Could you check a few things on this model? Use its own coordinates, in mm. Face numbers are marked on the shaded views. A direction names the side the tool comes from. Round coordinates to 2 decimals unless told otherwise and drop trailing zeros. Loops run counter-clockwise (first coordinate to the right, second up) from the corner with the lowest first, then second, coordinate; pieces in that order, holes last. Notation, with made-up numbers: (45.5, 53) -> (96.5, 53) arc R20 ccw to (96.5, 63) -> close; hole circle Ø3 at (-9, -22.5). An arc over 180 degrees is marked (long way). One line per item, written item: value.
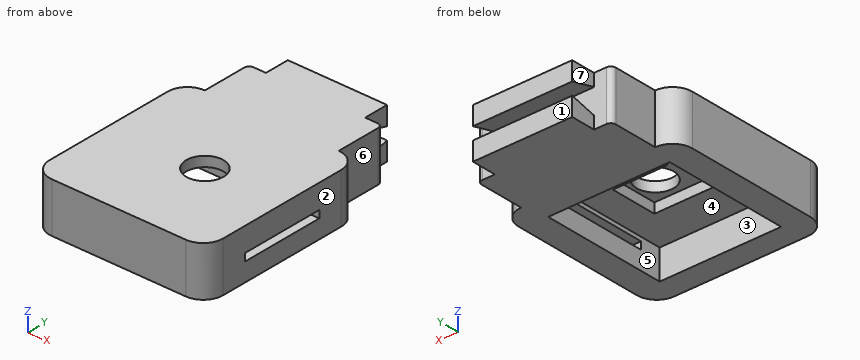
```python
from build123d import *

# Parameters (mm, degrees)
BOX_W           = 35
BOX_H           = 35
BOX_DEPTH       = 10
SKETCH_W        = 24.5
SKETCH_H        = 25.5
POCKET_DEPTH    = 8
SKETCH001_R     = 3.75
POCKET001_DEPTH = 2
PAD_DEPTH       = 2
SKETCH003_W     = 17
SKETCH003_H     = 1.5
POCKET002_DEPTH = 5.251
FILLET_R        = 4
FILLET_FACE7_W  = 27
FILLET_FACE7_H  = 10
PAD001_DEPTH    = 10
PAD001_FACE19_W = 27
PAD001_FACE19_H = 10
PAD002_DEPTH    = 5
POCKET003_DEPTH = 31.001
POCKET004_DEPTH = 3.5
POCKET005_DEPTH = 3.5
FILLET001_R     = 1


with BuildPart() as part:
    # Box → Box (new body)
    with BuildSketch(Plane.XY):
        with Locations((17.5, 17.5)):
            Rectangle(BOX_W, BOX_H)
    extrude(amount=BOX_DEPTH)

    # Sketch (on Face5 of BaseFeature) → Pocket (cut)
    with BuildSketch(Plane(origin=(0, 0, 0), x_dir=(1, 0, 0), z_dir=(0, 0, -1))):
        with Locations((17.5, -17.5)):
            Rectangle(SKETCH_W, SKETCH_H)
    extrude(amount=-POCKET_DEPTH, mode=Mode.SUBTRACT)

    # Sketch001 (on Face3 of Pocket) → Pocket001 (cut)
    with BuildSketch(Plane.XY.offset(10)):
        with Locations((19.25, 17.7)):
            Circle(SKETCH001_R)
    extrude(amount=-POCKET001_DEPTH, mode=Mode.SUBTRACT)

    # Sketch002 (on Face12 of Pocket001) → Pad (join)
    with BuildSketch(Plane(origin=(0, 0, 8), x_dir=(1, 0, 0), z_dir=(0, 0, -1))):
        Polygon((12.75, -30.25), (29.75, -30.25), (29.75, -4.75), (5.25, -4.75), (5.25, -12.75), (23.75, -12.75), (23.75, -22.25), (12.75, -22.25), align=None)
    extrude(amount=PAD_DEPTH)

    # Sketch003 (on Face9 of Pad) → Pocket002 (cut, through all)
    with BuildSketch(Plane(origin=(29.75, 0, 0), x_dir=(0, -1, 0), z_dir=(-1, 0, 0))):
        with Locations((-17.5, 4.45)):
            Rectangle(SKETCH003_W, SKETCH003_H)
    extrude(amount=-POCKET002_DEPTH, mode=Mode.SUBTRACT)

    # Fillet
    fillet_edges = [part.edges().sort_by_distance(p)[0] for p in [
        (0, 0, 5),
        (35, 0, 5),
        (0, 35, 5),
        (35, 35, 5),
    ]]
    fillet(fillet_edges, radius=FILLET_R)

    # Fillet Face7 → Pad001 (add)
    with BuildSketch(Plane(origin=(17.5, 35, 5), x_dir=(1, 0, 0), z_dir=(0, 1, 0))):
        Rectangle(FILLET_FACE7_W, FILLET_FACE7_H)
    extrude(amount=PAD001_DEPTH)

    # Pad001 Face19 → Pad002 (add)
    with BuildSketch(Plane(origin=(17.5, 45, 5), x_dir=(1, 0, 0), z_dir=(0, 1, 0))):
        Rectangle(PAD001_FACE19_W, PAD001_FACE19_H)
    extrude(amount=PAD002_DEPTH)

    # Sketch004 (on Face30 of Pad002) → Pocket003 (cut, through all)
    with BuildSketch(Plane.YZ.offset(31)):
        Polygon((45, 2.5), (45, 7.5), (50, 6.25), (50, 3.75), align=None)
    extrude(amount=-POCKET003_DEPTH, mode=Mode.SUBTRACT)

    # Sketch005 (on Face32 of Pocket003) → Pocket004 (cut)
    with BuildSketch(Plane.YZ.offset(31)):
        Polygon((45, 0), (45, 2.5), (50, 3.75), (50, 0), align=None)
        Polygon((45, 7.5), (45, 10), (50, 10), (50, 6.25), align=None)
    extrude(amount=-POCKET004_DEPTH, mode=Mode.SUBTRACT)

    # Sketch006 (on Face28 of Pocket004) → Pocket005 (cut)
    with BuildSketch(Plane(origin=(4, 0, 0), x_dir=(0, -1, 0), z_dir=(-1, 0, 0))):
        Polygon((-45, 10), (-45, 7.5), (-50, 6.25), (-50, 10), align=None)
        Polygon((-50, 3.75), (-50, 0), (-45, 0), (-45, 2.5), align=None)
    extrude(amount=-POCKET005_DEPTH, mode=Mode.SUBTRACT)

    # Fillet001
    fillet001_edges = [part.edges().sort_by_distance(p)[0] for p in [
        (4, 45, 5),
        (4, 45, 1.25),
        (4, 45, 8.75),
        (31, 45, 1.25),
        (31, 45, 5),
        (31, 45, 8.75),
    ]]
    fillet(fillet001_edges, radius=FILLET001_R)


solid = part.part
```
Item 1: If we mould it in two halves opening along X, with no side actions, what happens to the marked faces 1, 2, 3 and 4? For each: released by +X, released by -X, zero draft, split by the parting line, or undercut.
Output:
face 1: zero draft
face 2: released by +X
face 3: undercut
face 4: undercut
Item 2: For the marked faces 5, 6 and 7, which set-ups out of +Z, -Z, +X, -X, +Y, -Y let a thin tool reach every point of the face, with its end or its side?
Output:
face 5: -Z
face 6: +Z, -Z, +X, +Y
face 7: +Z, -Z, -X, +Y
Item 3: I need wall thicknesses on line 1 (Y direction, x = 19.25, z = 9.2); line 2 (Y direction, x = 28.5, z = 3.5); line 3 (X direction, y = 25, z = 1). Which ranges of each line are inside material? Lowest first, please. Write a range as from..to.
Output:
line 1: y = 0..13.95, 21.45..50
line 2: y = 0..4.75, 30.25..45
line 3: x = 0..5.25, 29.75..35
Item 4: Will these pins go through, and if not, where does the flat tip stop? pin 1 Ø1 at (x, y) = (26.5, 16.5) entering from -Z; pin 2 Ø1.9 at (y, z) = (46.5, 9) entering from +X; pin 3 Ø1.2 at (x, z) = (32.5, 4.5) entering from +Y.
Output:
pin 1: stops at z = 6
pin 2: stops at x = 27.5
pin 3: stops at y = 34.9
Item 5: If we section it at C-C on z = 1.5: List the corners of the cut face in (x, y) for me, plus the area to 3 significant figures.
Output:
outline: (0, 4) arc R4 ccw to (4, 0) -> (31, 0) arc R4 ccw to (35, 4) -> (35, 31) arc R4 ccw to (31, 35) -> (31, 44) arc R1 ccw to (30, 45) -> (27.5, 45) -> (27.5, 50) -> (7.5, 50) -> (7.5, 45) -> (5, 45) arc R1 ccw to (4, 44) -> (4, 35) arc R4 ccw to (0, 31) -> close; hole (5.25, 4.75) -> (29.75, 4.75) -> (29.75, 30.25) -> (5.25, 30.25) -> close
area: 956 mm²
Item 6: If we section it at B-B on x = 19.25: List the corners of the cut face in (y, z) for me, plus the area to 3 significant figures.
Output:
outline: (0, 0) -> (4.75, 0) -> (4.75, 6) -> (12.75, 6) -> (12.75, 8) -> (13.95, 8) -> (13.95, 10) -> (0, 10) -> close; (21.45, 8) -> (22.25, 8) -> (22.25, 6) -> (30.25, 6) -> (30.25, 0) -> (50, 0) -> (50, 3.75) -> (45, 2.5) -> (45, 7.5) -> (50, 6.25) -> (50, 10) -> (21.45, 10) -> close
area: 294 mm²
Item 7: If we section it at D-D on y = 11: List the corners of the cut face in (x, z) for me, plus the area to 3 significant figures.
Output:
outline: (0, 0) -> (5.25, 0) -> (5.25, 6) -> (29.75, 6) -> (29.75, 5.2) -> (35, 5.2) -> (35, 10) -> (0, 10) -> close; (29.75, 0) -> (35, 0) -> (35, 3.7) -> (29.75, 3.7) -> close
area: 195 mm²
Item 8: If we section it at A-A on y = 17.7: List the corners of the cut face in (x, z) for me.
Output:
outline: (0, 0) -> (5.25, 0) -> (5.25, 8) -> (15.5, 8) -> (15.5, 10) -> (0, 10) -> close; (23, 8) -> (23.75, 8) -> (23.75, 6) -> (29.75, 6) -> (29.75, 5.2) -> (35, 5.2) -> (35, 10) -> (23, 10) -> close; (29.75, 0) -> (35, 0) -> (35, 3.7) -> (29.75, 3.7) -> close
